For this review, use the dimensioned drawing (mm, ordinates from the lowest corner) and the shaded views. Give positions to 0.01 mm unless a question says otherwise; leave off trailing zeros. Write each loop counter-clockwise with the first axis right and the second up, starting at its lowest first coordinate (ties: lowest second). Pieces come first, ordered by that corner, then holes. Notation, with made-up numbers: M -16.5,-25.75 L 18.5,-25.75 A23 cw 18.5,12.25 Z; hole C 8,-34 d7. An arc over 180 degrees is marked long. Write each question's results on one line, items separated by ' | '. Start each with the question number.
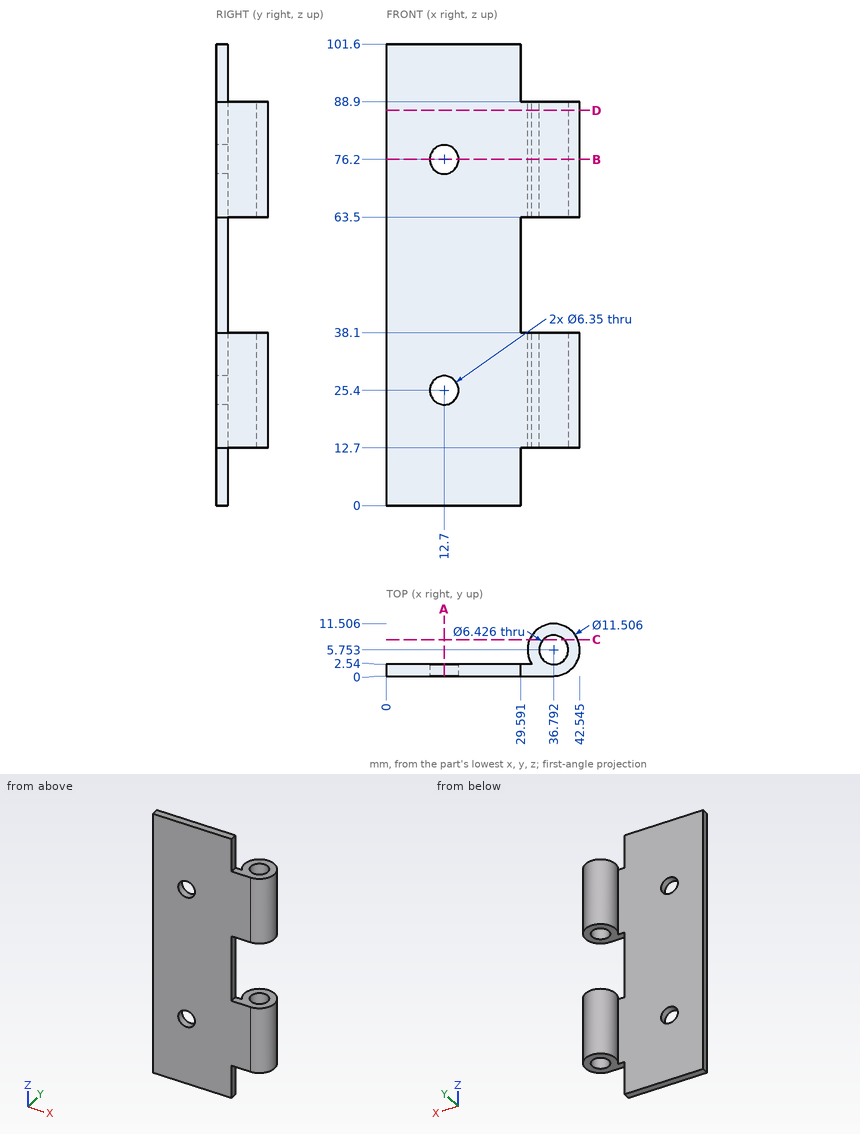
(1) Add section D-D (z = 87). State the section outline as (x, y) points (1 decimal).
(2) Add section B-B (z = 76.2). State the section outline as (x, y) points (1 decimal).
(3) Add section A-A (x = 12.7). State the section outline as (y, z) points (3 decimals), then the cut area to 3 significant figures.
(4) Wall thickness on L1, parallel to Z at x = 12.7, y = 1.35 (3 decimals); L2, parallel to X at y = 5.75, z = 70.5 (1 decimal); L3, parallel to Z at x = 40, y = 10.25: over which ranges is each line inside the solid? List them lowest first.
(5) Add section C-C (y = 8). State the section outline as (x, z) points (1 decimal), then the cut area to 3 significant figures.
(6) Clearance check with flat-ended pins moving along their axes: P1, Ø10, axis at x = 12.7, z = 76.2, coming from the +Y side; P2, Ø2, axis at y = 1.5, z = 98, coming from the +X side; P3, Ø6, axis at x = 34.5, y = 6, coming from the -Z side; P4, Ø6, axis at x = 36.79, y = 5.75, coming from the +Z side. State where each tip first meets the part, or that it passes through.
Calculated:
1) outline: M 0,0 L 36.8,0 A5.8 ccw long 32,2.5 L 0,2.5 Z; hole C 36.8,5.8 d6.4
2) outline: M 0,0 L 9.5,0 L 9.5,2.5 L 0,2.5 Z; M 15.9,0 L 36.8,0 A5.8 ccw long 32,2.5 L 15.9,2.5 Z; hole C 36.8,5.8 d6.4
3) outline: M 0,0 L 2.54,0 L 2.54,22.225 L 0,22.225 Z; M 0,28.575 L 2.54,28.575 L 2.54,73.025 L 0,73.025 Z; M 0,79.375 L 2.54,79.375 L 2.54,101.6 L 0,101.6 Z | area: 226 mm²
4) L1: z = 0 to 22.225, 28.575 to 73.025, 79.375 to 101.6 | L2: x = 31 to 33.6, 40 to 42.5 | L3: z = 12.7 to 38.1, 63.5 to 88.9
5) outline: M 31.5,12.7 L 34.5,12.7 L 34.5,38.1 L 31.5,38.1 Z; M 31.5,63.5 L 34.5,63.5 L 34.5,88.9 L 31.5,88.9 Z; M 39.1,12.7 L 42.1,12.7 L 42.1,38.1 L 39.1,38.1 Z; M 39.1,63.5 L 42.1,63.5 L 42.1,88.9 L 39.1,88.9 Z | area: 305 mm²
6) P1: stops at y = 2.54 | P2: stops at x = 29.59 | P3: stops at z = 12.7 | P4: passes through
